```python
from build123d import *

# Parameters (mm, degrees)
F0_R         = 11.1
F1_DEPTH     = 150
F2_W         = 22.5644709975
F2_H         = 75
F4_DEPTH     = 7.5
F5_W         = 300
F5_H         = 100
F5_W_2       = 15
F5_H_2       = 22.5644709975
F7_DEPTH     = 10
F8_SIZE2     = 50
F8_SIZE      = 10
F9_T4_ANGLE  = 180
F9_T10_ANGLE = 180


# Not quite as in the source:
# - a fillet or chamfer that OpenCascade refuses, or shapes differently, is made with other operations: its cross-section is extruded or revolved along the edge and cut away or added


with BuildPart() as f1:
    # F0 (on Right) → F1 (new body, symmetric)
    with BuildSketch(Plane.YZ):
        Circle(F0_R)
    extrude(amount=F1_DEPTH, both=True)

    # F2 (on Right) → F4 (join, symmetric)
    with BuildSketch(Plane.YZ):
        with Locations((-0.1822354987, -37.5)):
            Rectangle(F2_W, F2_H)
    extrude(amount=F4_DEPTH, both=True)

    # F6: fillet of radius 2 on 2 edges, made by hand

    # F6_s1 → F6_t2 (revolve, cut)
    with BuildSketch(Plane.XY):
        with BuildLine():
            ThreePointArc((-148, 11.1), (-149.4142135624, 10.5142135624), (-150, 9.1))
            Line((-150, 9.1), (-150, 11.1))
            Line((-150, 11.1), (-148, 11.1))
        make_face()
    revolve(axis=Axis((-150, 0, 0), (1, 0, 0)), mode=Mode.SUBTRACT)

    # F6_s3 → F6_t4 (revolve, cut)
    with BuildSketch(Plane.XY):
        with BuildLine():
            ThreePointArc((148, 11.1), (149.4142135624, 10.5142135624), (150, 9.1))
            Line((150, 9.1), (150, 11.1))
            Line((150, 11.1), (148, 11.1))
        make_face()
    revolve(axis=Axis((150, 0, 0), (1, 0, 0)), mode=Mode.SUBTRACT)

    # F5 (on face) → F7 (join)
    with BuildSketch(Plane(origin=(0, 0, -75), x_dir=(1, 0, 0), z_dir=(0, 0, -1))):
        Rectangle(F5_W, F5_H)
        with Locations((0, 0.1822354987)):
            Rectangle(F5_W_2, F5_H_2, mode=Mode.SUBTRACT)
    extrude(amount=-F7_DEPTH)

    # F8
    f8_edges = [f1.edges().sort_by_distance(p)[0] for p in [
        (7.5, -0.182235, -65),
        (0, -11.464471, -65),
        (0, 11.1, -65),
        (-7.5, -0.182235, -65),
    ]]
    f8_side = f1.faces().sort_by_distance((146.837722, 0, -65))[0]
    chamfer(f8_edges, length=F8_SIZE, length2=F8_SIZE2, reference=f8_side)

    # F9: fillet of radius 10 on 2 edges, made by hand


with BuildPart() as f9_tool2:
    # F9_s3 → F9_t4 (revolve)
    with BuildSketch(Plane.XY):
        with BuildLine():
            ThreePointArc((7.5, -21.1), (10.4289321881, -14.0289321881), (17.5, -11.1))
            Line((17.5, -11.1), (7.5, -11.1))
            Line((7.5, -11.1), (7.5, -21.1))
        make_face()
    revolve(axis=Axis((7.5, 0, 0), (1, 0, 0)), revolution_arc=F9_T4_ANGLE)

    split(bisect_by=Plane.XZ.offset(-11.1), keep=Keep.TOP)

    split(bisect_by=Plane.XZ.offset(11.4644709975), keep=Keep.BOTTOM)


with BuildPart() as f1_1:
    add(f1.part)

    # F9_t1: union F9_tool2
    add(f9_tool2.part)


with BuildPart() as f9_tool8:
    # F9_s9 → F9_t10 (revolve)
    with BuildSketch(Plane.XY):
        with BuildLine():
            ThreePointArc((-17.5, -11.1), (-10.4289321881, -14.0289321881), (-7.5, -21.1))
            Line((-7.5, -21.1), (-7.5, -11.1))
            Line((-7.5, -11.1), (-17.5, -11.1))
        make_face()
    revolve(axis=Axis((-7.5, 0, 0), (1, 0, 0)), revolution_arc=F9_T10_ANGLE)

    split(bisect_by=Plane.XZ.offset(-11.1), keep=Keep.TOP)

    split(bisect_by=Plane.XZ.offset(11.4644709975), keep=Keep.BOTTOM)


with BuildPart() as f1_2:
    add(f1_1.part)

    # F9_t7: union F9_tool8
    add(f9_tool8.part)


solid = f1_2.part
```
The model under review builds one solid part; all positions refer to its coordinate system, in mm. A direction names the side the tool comes from. Round coordinates to 2 decimals unless told otherwise and drop trailing zeros. Loops run counter-clockwise (first coordinate to the right, second up) from the corner with the lowest first, then second, coordinate; pieces in that order, holes last. Notation, with made-up numbers: M -16.5,-40 L 6.5,-40 A24 cw 6.5,-1 Z; hole C -38.75,58.25 d11. An arc over 180 degrees is marked long. Write item = value, one per line.
Item 1: Take a section at D-D on z = -42. Write out the cut boundary in (x, y).
Return value:
outline = M -12.9,-16.86 L 12.9,-16.86 L 12.9,16.5 L -12.9,16.5 Z
Item 2: The part is to be moulded in two halves that separate along Z. For faces 1 (the flat face through (-13.54, 0.12, -45.21)), 2 (the flat face through (-0.245, -17.506, -45.206)), 3 (the flat face through (-150, 0, 0)), 4 (the flat face through (-2, -1, -75)), say which applies: released by +Z, released by -Z, zero draft, split by the parting line, or undercut.
Return value:
face_1 = undercut
face_2 = released by +Z
face_3 = zero draft
face_4 = released by -Z
Item 3: For line 1 (Z direction, x = -19, y = -0.5); line 2 (Z direction, x = -106.5, y = -42); line 3 (Y direction, x = 49, z = 1.5), list the stretches that pass through material, from the lowest coordinate up. Write a range as [from, to].
Return value:
line_1 = [-75, -65], [-11.09, 11.09]
line_2 = [-75, -65]
line_3 = [-11, 11]
Item 4: Machinability: for faces 5 (the flat face through (0, -11.464, -6)), 6 (the flat face through (-2, 50, -70)), 7 (the cylindrical face through (2.072, -1.445, 11.006)), 8 (the flat face through (0, 11.1, -6)), which of the approach directions +Z, -Z, +X, -X, +Y, -Y give a long, thin tool a straight path to every point of the face, cutting with its end or side? Answer none if there is none.
Return value:
face_5 = +Z, +X, -X, -Y
face_6 = +Z, -Z, +X, -X, +Y
face_7 = none
face_8 = +Z, +X, -X, +Y
Item 5: Take a section at A-A on x = 95. Write out the cut boundary in (y, z).
Return value:
outline = M -50,-75 L 50,-75 L 50,-65 L -50,-65 Z; C 0,0 d22.2
Item 6: Insertion check: P1, Ø4.5, axis at x = 0.5, z = -8, coming from the -Y side; P2, Ø17.5, axis at x = -2.5, z = -10.5, coming from the +Y side; P3, Ø1, axis at y = -3.5, z = -31, coming from the -X side. Each pin has a flat end and moves straight along its axis. Give the tip position at first contact, or say it passes through.
Return value:
P1 = -11.46
P2 = 11.95
P3 = -10.8
Item 7: Take a section at B-B on y = 18. Write out the cut boundary in (x, z), then the cut area to 3 significant figures.
Return value:
outline = M -150,-75 L 150,-75 L 150,-65 L 17.5,-65 L 14.4,-49.5 L -14.4,-49.5 L -17.5,-65 L -150,-65 Z
area = 3,490 mm2
Item 8: Take a section at C-C on y = -17.5. Write out the cut boundary in (x, z), then the cut area to 3 significant figures.
Return value:
outline = M -150,-75 L 150,-75 L 150,-65 L 17.5,-65 L 13.54,-45.18 L -13.54,-45.18 L -17.5,-65 L -150,-65 Z
area = 3,620 mm2
